from build123d import *

# Parameters (mm, degrees)
FILLET_1_R          = 0.5
SKETCH_2_R          = 12.5
CUT_EXTRUDE_1_DEPTH = 0.5


with BuildPart() as part:
    # Эскиз1 → Повернуть1 (revolve)
    with BuildSketch(Plane(origin=(0, 0, 0), x_dir=(1, 0, 0), z_dir=(0, 1, 0))):
        Polygon((0, 0), (-32, 0), (-32, 4), (-35, 4), (-35, 19), (-32, 19), (-32, 23), (0, 23), align=None)
    revolve(axis=Axis((0, 0, -23), (0, 0, 1)))

    # Скругление1
    fillet_1_edges = [part.edges().sort_by_distance(p)[0] for p in [
        (32, 0, -23),
        (32, 0, 0),
    ]]
    fillet(fillet_1_edges, radius=FILLET_1_R)

    # Эскиз2 → Вырез-Вытянуть1 (cut)
    with BuildSketch(Plane(origin=(0, 0, -23), x_dir=(-1, 0, 0), z_dir=(0, 0, -1))):
        Circle(SKETCH_2_R)
    extrude(amount=-CUT_EXTRUDE_1_DEPTH, mode=Mode.SUBTRACT)

    # Эскиз3 → Вырез-Повернуть1 (revolve, cut)
    with BuildSketch(Plane(origin=(0, 0, 0), x_dir=(0, 0, -1), z_dir=(1, 0, 0)), mode=Mode.PRIVATE) as cut_revolve_1_sk:
        Polygon((22.5, 0), (19.5, 0), (22.5, 3), align=None)
    revolve(cut_revolve_1_sk.sketch.rotate(Axis((0, 0, -22.5), (0, 0, 1)), 270), axis=Axis((0, 0, -22.5), (0, 0, 1)), mode=Mode.SUBTRACT)


solid = part.part
Input: part model. Units: mm. Frame: model coordinates. A direction names the side the tool comes from. Coordinates: 2 decimals unless noted, no trailing zeros. Order: outer loops, then holes, each group sorted by start corner. A loop starts at its lowest first (then second) coordinate and runs counter-clockwise, first axis right, second up. Notation, with made-up numbers: M -13.5,-21.75 L 5.5,-21.75 A27 cw 5.5,5.25 Z; hole C -35,48.25 d6. An arc over 180 degrees is marked long. Answer in a Markdown table with one row per item.
(1) Draft query along X for faces 1 (the flat face through (-3, -3, -22.5)), 2 (the flat face through (15.4, 28.4, -4)), 3 (the cylindrical face through (6.94, 31.24, -20.77)). Return one class per face: pulls with the +X half, pulls with the -X half, needs draft (parallel to the pull), parting line crosses it, or undercut.
Numbers:
| item | result |
|---|---|
| face 1 | undercut |
| face 2 | needs draft |
| face 3 | parting line crosses it |
(2) Contact query for flat-ended pins moving along their axis: pin 1 Ø3 at (y, z) = (15, -18.5) entering from -X; pin 2 Ø4 at (x, z) = (-23, -9.5) entering from -Y; pin 3 Ø12.5 at (x, y) = (-3.5, 3) entering from -Z. Output: stop coordinate, or through.
Numbers:
| item | result |
|---|---|
| pin 1 | stops at x = -32.29 |
| pin 2 | stops at y = -28 |
| pin 3 | stops at z = -22.5 |
(3) Access query for faces 4 (the cylindrical face through (6.94, 31.24, -2.27)), 5 (the flat face through (-14, 0, -23)), 6 (the flat face through (-15.4, 28.4, -19)). Directions: +Z, -Z, +X, -X, +Y, -Y. A direction counts if a zero-diameter tool reaches every point of the face in a straight line with its end or side. Return the directions, or none.
Numbers:
| item | result |
|---|---|
| face 4 | +Z |
| face 5 | -Z, +X, -X, +Y, -Y |
| face 6 | -Z |
(4) Section query A-A, the plane z = -15.25. Output: boundary loops of the cut face in (x, y), plus the area to 3 significant figures.
Numbers:
| item | result |
|---|---|
| outline | C 0,0 d70 |
| area | 3,850 mm^2 |
(5) Material intervals for line 1 (Y direction, x = 0, z = -22.55); line 2 (Z direction, x = -9, y = 32); line 3 (Z direction, x = -4.5, y = 0), sorted ascending. Write a range as [from, to].
Numbers:
| item | result |
|---|---|
| line 1 | y = [-32, -12.5], [12.5, 32] |
| line 2 | z = [-19, -4] |
| line 3 | z = [-22.5, 0] |
